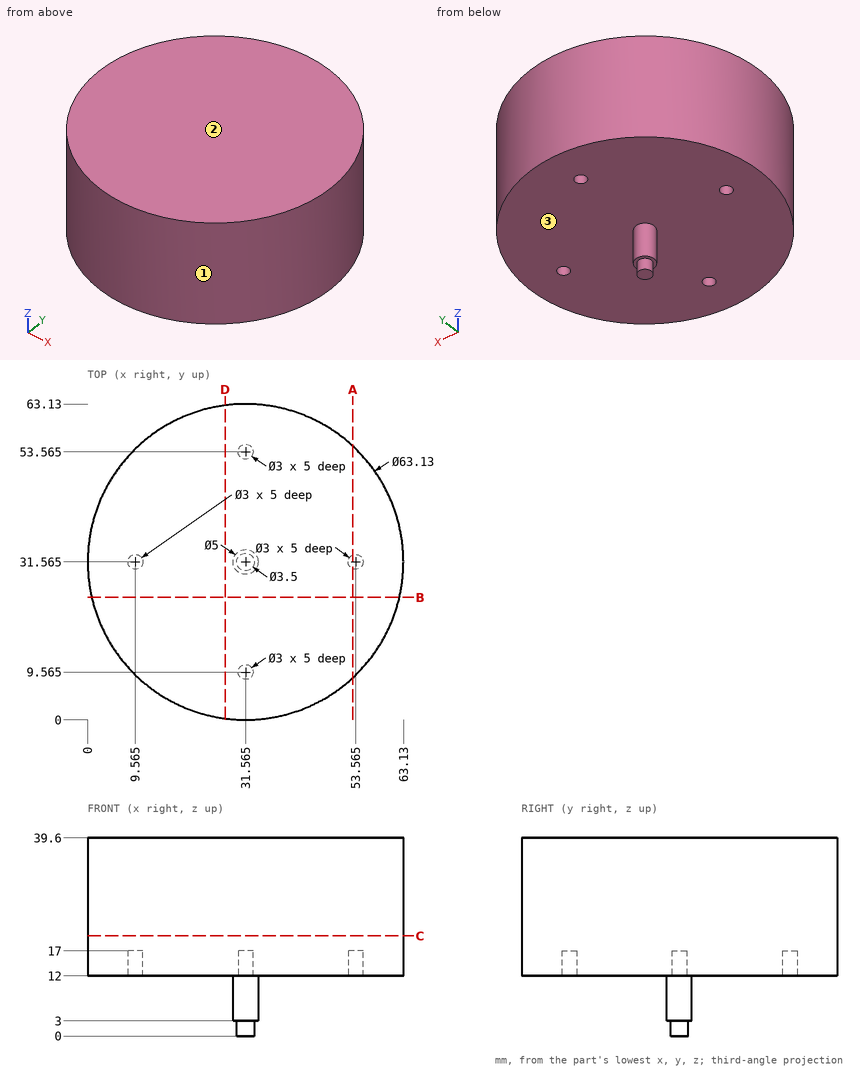
Source: three-view drawing plus pictorial views. Frame: mm from the lowest corner of the part. Coordinates: 2 decimals unless noted, no trailing zeros. Loops run counter-clockwise (first coordinate to the right, second up) from the corner with the lowest first, then second, coordinate; pieces in that order, holes last. Notation, with made-up numbers: (68, 52) -> (100, 52) arc R17 cw to (100, 84) -> close; hole circle Ø1 at (-22.75, 68.5). An arc over 180 degrees is marked (long way). Answer in a Markdown table with one row per item. Add a question column.
Q1. Section A-A on x = 53. Return the cut outline in (y, z), and give its area (3 significant figures).
Q2. Pull-direction query (Z, two-part tool) for the marked faces 1, 2 and 3; classes: pulls with the +Z half, pulls with the -Z half, needs draft (parallel to the pull), parting line crosses it, or undercut.
Q3. Ray query, line 1 along Z through (x, y) = (48.5, 12); line 2 along X through (y, z) = (31.5, 11); line 3 along Y through (x, z) = (15.5, 24). Return the intervals inside material, ascending.
Q4. Section C-C on z = 20. Return the cut outline in (x, y) (3 decimals), and give its area (3 significant figures).
Q5. Contact query for flat-ended pins moving along their axis: pin 1 Ø1 at (x, z) = (21, 12) entering from -Y; pin 2 Ø4 at (x, z) = (38, 25) entering from +Y; pin 3 Ø8 at (y, z) = (41, 13) entering from -X; pin 4 Ø19 at (x, y) = (31.5, 23) entering from -Z. Output: stop coordinate, or through.
Q6. Section D-D on x = 27.5. Return the cut outline in (y, z).
Q7. Section B-B on y = 24.5. Return the cut outline in (x, z).
Computed values:
| question | item | result |
|---|---|---|
| 1 | outline | (8.39, 12) -> (30.18, 12) -> (30.18, 17) -> (32.95, 17) -> (32.95, 12) -> (54.74, 12) -> (54.74, 39.6) -> (8.39, 39.6) -> close |
| 1 | area | 1,270 mm^2 |
| 2 | face 1 | needs draft |
| 2 | face 2 | pulls with the +Z half |
| 2 | face 3 | pulls with the -Z half |
| 3 | line 1 | z = 12 to 39.6 |
| 3 | line 2 | x = 29.07 to 34.06 |
| 3 | line 3 | y = 4.39 to 58.74 |
| 4 | outline | circle Ø63.13 at (31.565, 31.565) |
| 4 | area | 3,130 mm^2 |
| 5 | pin 1 | stops at y = 1.65 |
| 5 | pin 2 | stops at y = 62.82 |
| 5 | pin 3 | stops at x = 0.47 |
| 5 | pin 4 | stops at z = 0 |
| 6 | outline | (0.26, 12) -> (62.87, 12) -> (62.87, 39.6) -> (0.26, 39.6) -> close |
| 7 | outline | (0.8, 12) -> (62.33, 12) -> (62.33, 39.6) -> (0.8, 39.6) -> close |
